Autodesk Inventor part; units mm, degrees
ref_plane "Work Plane1" through (-24.1297, -20.1241, 6.985) normal (0, 0, -1) x (0, 1, 0)
ref_plane "Work Plane2" through (-24.1297, -20.1241, 10.16) normal (0, 0, 1) x (1, 0, 0)
ref_plane "Work Plane4" through (-33.6547, -38.1116, -58.8269) normal (-1, 0, 0) x (0, 0.0012, 1)
sketch "Sketch1" plane through (0, 0, 0) normal (0, 0, 1) x (1, 0, 0)
  circle A0 centre (0, 0) radius 14
  arc A1 (-9.6844, 3.0721) -> (-9.6844, -3.0721) centre (0, 0) ccw construction
  circle A2 centre (0, 0) radius 14
ref_plane "Work Plane1" through (-24.1297, -20.1241, 6.985) normal (0, 0, -1) x (0, 1, 0)
extrude "Extrusion1" add sketch "Sketch1" along normal up to surface (6.985 mm away)
sketch "Sketch2" plane through (0, 0, 6.985) normal (0, 0, 1) x (1, 0, 0)
  line L0 (24.1297, -19.05) -> (-24.1297, -19.05) construction
  line L1 (30.4797, -4.9571) -> (30.4797, -51.5313) construction
  line L2 (-30.4797, -51.5313) -> (-30.4797, -4.9571) construction
  line L3 (-6.5797, 18.2867) -> (-30.4797, 3.81)
  line L4 (6.5797, 18.2867) -> (30.4797, 3.81)
  line L5 (30.4797, 3.81) -> (30.4797, -19.05)
  line L6 (30.4797, -19.05) -> (-30.4797, -19.05)
  line L7 (-30.4797, -19.05) -> (-30.4797, 3.81)
  line L8 (0, 141.501) -> (0, -68.047)
  arc A0 (6.5797, 18.2867) -> (-6.5797, 18.2867) centre (0, 7.4241) ccw construction
  line L9 (6.5797, 18.2867) -> (24.1297, 7.6563) construction
  line L10 (-24.1297, 7.6563) -> (-6.5797, 18.2867) construction
  line L11 (6.5797, 18.2867) -> (-6.5797, 18.2867)
  point P0 (0, 0)
  point P1 (0, -5.2759)
  point P2 (-30.4797, 16.6942)
  point P3 (-5.3196, -19.05)
ref_plane "Work Plane2" through (-24.1297, -20.1241, 10.16) normal (0, 0, 1) x (1, 0, 0)
extrude "Extrusion2" add sketch "Sketch2" along normal up to surface (3.175 mm away)
ref_plane "Work Plane3" through (30.4797, -27.7824, 45.9277) normal (-1, 0, 0) x (0, -0.986, 0.1668)
sketch "Sketch3" plane through (30.4797, -27.7824, 45.9277) normal (-1, 0, 0) x (0, -0.986, 0.1668)
  line L0 (-47.9068, 72.7646) -> (-31.8636, 83.3523) construction
  line L1 (-25.5087, 83.7046) -> (-20.9193, 81.3584) construction
  line L2 (-17.4786, 75.8356) -> (-17.0001, 46.1314) construction
  line L3 (-61.535, 29.6482) -> (-50.5122, 69.1886) construction
  line L4 (-45.3902, -22.2294) -> (-61.4405, 25.9552) construction
  line L5 (-15.9257, 42.7078) -> (21.8176, -13.4116) construction
  line L6 (24.78, -27.1582) -> (21.9473, -43.9057) construction
  line L7 (-18.293, -38.7417) -> (-32.0753, -36.4163) construction
  line L8 (-35.8826, -34.2371) -> (-44.4025, -24.0864) construction
  line L9 (1.5345, -78.0839) -> (-13.5009, -42.5299) construction
  line L10 (52.2811, -114.2632) -> (3.7676, -80.8246) construction
  line L11 (22.2253, -47.0922) -> (25.3496, -55.8788) construction
  line L12 (27.7289, -58.9798) -> (55.688, -78.2509) construction
  line L13 (58.1761, -81.7138) -> (65.2363, -106.3801) construction
  line L14 (60.9015, -114.1914) -> (57.6044, -115.1351) construction
  line L15 (-49.878, 71.4637) -> (-28.7889, 85.3815)
  line L16 (-28.7889, 85.3815) -> (-17.5398, 79.6307)
  line L17 (-17.5398, 79.6307) -> (-16.9699, 44.2605)
  line L18 (-16.9699, 44.2605) -> (26.0426, -19.6937)
  line L19 (26.0426, -19.6937) -> (21.6717, -45.5351)
  line L20 (21.6717, -45.5351) -> (26.0378, -57.8141)
  line L21 (26.0378, -57.8141) -> (57.5529, -79.5363)
  line L22 (57.5529, -79.5363) -> (66.9746, -112.4531)
  line L23 (66.9746, -112.4531) -> (54.7369, -115.9559)
  line L24 (54.7369, -115.9559) -> (2.2516, -79.7797)
  line L25 (2.2516, -79.7797) -> (-14.8578, -39.3213)
  line L26 (-14.8578, -39.3213) -> (-34.38, -36.0274)
  line L27 (-34.38, -36.0274) -> (-45.0145, -23.3573)
  line L28 (-45.0145, -23.3573) -> (-62.0524, 27.7923)
  line L29 (-62.0524, 27.7923) -> (-49.878, 71.4637)
  point P0 (-35.053, -40.651)
  point P1 (21.6748, -26.5696)
  point P2 (-49.9314, -21.2415)
  point P3 (-37.7332, 79.4786)
ref_plane "Work Plane4" through (-33.6547, -38.1116, -58.8269) normal (-1, 0, 0) x (0, 0.0012, 1)
extrude "Extrusion4" add sketch "Sketch3" against normal blind 4
mirror "Mirror1" about plane through (0, 0, 0) normal (1, 0, 0) of "Extrusion4"
properties part number "ShoulderCollision"
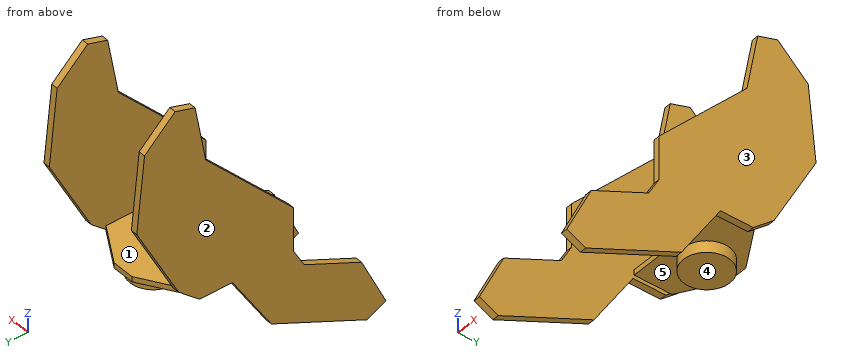
Can you work these out from the model? Positions are in its coordinate system, mm. Face numbers are marked on the shaded views. A direction names the side the tool comes from. Give positions to 0.01 mm unless a question says otherwise; leave off trailing zeros. Loops run counter-clockwise (first coordinate to the right, second up) from the corner with the lowest first, then second, coordinate; pieces in that order, holes last. Notation, with made-up numbers: M 45.5,87 L 93.5,87 A27 cw 93.5,110 Z; hole C 24,-31.75 d2. An arc over 180 degrees is marked long. Use one line per item in the form item = value. Start each with the question number.
(1) I want a section at D-D, the plane x = 21.5. Write out the boundary of the cut face in (y, z) (3 decimals), and give its area (4 significant figures).
(2) Please list where these lines run through material, in increasing order: line 1 (X direction, y = 1, z = 79); line 2 (Z direction, x = -24, y = -6.5) (3 decimals); line 3 (Y direction, x = -31, z = -30.5).
(3) I'm going to push flat-ended pins straight in: P1, Ø14, axis at x = 7, y = 1.5, coming from the -Z side; P2, Ø8, axis at y = 6, z = 6, coming from the +X side; P3, Ø12, axis at x = -23.5, z = 69.5, coming from the +Y side; P4, Ø4.5, axis at x = -33, z = 19, coming from the -Y side. Where does each tip first touch, or does it pass through?
(4) I want a section at A-A, the plane z = 24.5. Write out the boundary of the cut face in (x, y).
(5) I want a section at B-B, the plane y = -38.5. Write out the boundary of the cut face in (x, z).
(6) Thinking about a two-plate mould opening in X: for the marked faces 3, 4 and 5, which applies, released by +X, released by -X, zero draft, split by the parting line, or undercut?
(7) I want a section at C-C, the plane x = 0. Write out the boundary of the cut face in (y, z) (3 decimals).
(8) On a 3-axis mill with a long thin cutter (end or side, diameter ignored), from which of +Z, -Z, +X, -X, +Y, -Y can I reach the whole of each face in a straight line? I mean the marked faces 1 and 2. Say none if no direction works.
Worked out:
q1.outline = M -19.05,6.985 L 9.249,6.985 L 9.249,10.16 L -19.05,10.16 Z
q1.area = 89.85 mm²
q2.line_1 = -34.48 to -30.48, 30.48 to 34.48
q2.line_2 = 6.985 to 10.16
q2.line_3 = -101.44 to -42.12
q3.P1 = 0
q3.P2 = 34.48
q3.P3 = through
q3.P4 = -56.75
q4.outline = M -34.48,-56.75 L -30.48,-56.75 L -30.48,17.55 L -34.48,17.55 Z; M 30.48,-56.75 L 34.48,-56.75 L 34.48,17.55 L 30.48,17.55 Z
q5.outline = M -34.48,-24.82 L -30.48,-24.82 L -30.48,50.06 L -34.48,50.06 Z; M 30.48,-24.82 L 34.48,-24.82 L 34.48,50.06 L 30.48,50.06 Z
q6.face_3 = released by +X
q6.face_4 = zero draft
q6.face_5 = undercut
q7.outline = M -19.05,6.985 L -14,6.985 L -14,0 L 14,0 L 14,6.985 L 18.287,6.985 L 18.287,10.16 L -19.05,10.16 Z
q8.face_1 = +Z, +Y, -Y
q8.face_2 = +Z, -Z, -X, +Y, -Y
